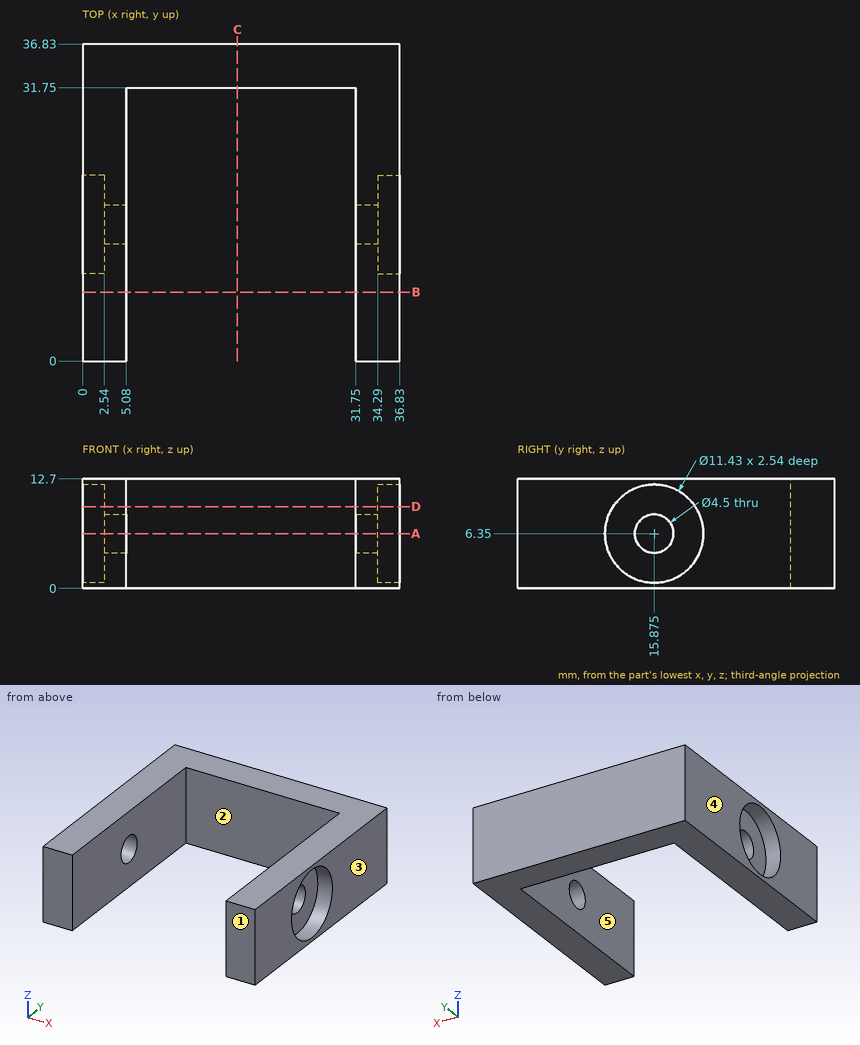
Print and shaded views of the part. All mm, measured from the part's lowest x, y and z. A direction names the side the tool comes from. Coordinates: 2 decimals unless noted, no trailing zeros. Loops run counter-clockwise (first coordinate to the right, second up) from the corner with the lowest first, then second, coordinate; pieces in that order, holes last. Notation, with made-up numbers: (89.5, 4.5) - (131.5, 4.5) arc R18 ccw to (131.5, 21.5) - close; hole circle Ø9 at (7.25, 29.25). An arc over 180 degrees is marked (long way). Write item = value, one per line. Start each with the question number.
Item 1: Saw through at D-D, the plane z = 9.5. List the corners of the cut face in (x, y).
Item 2: Saw through at C-C, the plane x = 18. List the corners of the cut face in (y, z), then the cut area to 3 significant figures.
Item 3: Pull direction X, two halves, no side cores. Call the marked faces 1, 2 and 3: +X half, -X half, draft (parallel to the pull), parting line (faces both ways), or undercut.
Item 4: 3-axis set-ups, long thin cutter, end or side, ignore diameter. For the marked faces 4 and 5: which of +Z, -Z, +X, -X, +Y, -Y reach the whole face in a straight line?
Item 5: Wall check: probe 1 along Y at (x, z) = (35.1, 6.35); probe 2 along X at (y, z) = (24, 4.5); probe 3 along Y at (x, z) = (33.1, 6.35) (3 decimals). Give the ranges that are in metal, low to high. Write a range as [from, to].
Item 6: Saw through at A-A, the plane z = 6.35. List the corners of the cut face in (x, y) (3 decimals), then the cut area to 3 significant figures.
Item 7: Drop flat-ended pins along their axis: pin 1 Ø4 at (y, z) = (15.5, 5) entering from -X; pin 2 Ø6.5 at (x, z) = (19, 4.5) entering from -Y; pin 3 Ø7 at (y, z) = (15.875, 6.35) entering from +X. Give the stop position or say it passes through.
Item 8: Saw through at B-B, the plane y = 8. List the corners of the cut face in (x, z).
Answers:
q1.outline = (0, 0) - (5.08, 0) - (5.08, 31.75) - (31.75, 31.75) - (31.75, 0) - (36.83, 0) - (36.83, 11.11) - (34.29, 11.11) - (34.29, 20.64) - (36.83, 20.64) - (36.83, 36.83) - (0, 36.83) - (0, 20.64) - (2.54, 20.64) - (2.54, 11.11) - (0, 11.11) - close
q2.outline = (31.75, 0) - (36.83, 0) - (36.83, 12.7) - (31.75, 12.7) - close
q2.area = 64.5 mm2
q3.face_1 = draft
q3.face_2 = undercut
q3.face_3 = +X half
q4.face_4 = +Z, -Z, -X, +Y, -Y
q4.face_5 = +Z, -Z, -Y
q5.probe_1 = [0, 10.16], [21.59, 36.83]
q5.probe_2 = [0, 5.08], [31.75, 36.83]
q5.probe_3 = [0, 13.625], [18.125, 36.83]
q6.outline = (0, 0) - (5.08, 0) - (5.08, 13.625) - (2.54, 13.625) - (2.54, 10.16) - (0, 10.16) - close; (0, 21.59) - (2.54, 21.59) - (2.54, 18.125) - (5.08, 18.125) - (5.08, 31.75) - (31.75, 31.75) - (31.75, 18.125) - (34.29, 18.125) - (34.29, 21.59) - (36.83, 21.59) - (36.83, 36.83) - (0, 36.83) - close; (31.75, 0) - (36.83, 0) - (36.83, 10.16) - (34.29, 10.16) - (34.29, 13.625) - (31.75, 13.625) - close
q6.area = 429 mm2
q7.pin_1 = 2.54
q7.pin_2 = 31.75
q7.pin_3 = 34.29
q8.outline = (0, 0) - (5.08, 0) - (5.08, 12.7) - (0, 12.7) - close; (31.75, 0) - (36.83, 0) - (36.83, 12.7) - (31.75, 12.7) - close
